Input: dimensioned drawing with shaded views. Units: mm. Origin: part minimum x, y, z. A direction names the side the tool comes from. Coordinates: 2 decimals unless noted, no trailing zeros. Loops run counter-clockwise (first coordinate to the right, second up) from the corner with the lowest first, then second, coordinate; pieces in that order, holes last.
Item 1: Line query: probe 1 along Z at (x, y) = (18.75, 20.5) (1 decimal); probe 2 along Y at (x, z) = (10.25, 5.5) (1 decimal); probe 3 along Z at (x, y) = (12.7, 1.4). Output: solid intervals per line, ascending.
Item 2: Section query B-B, the plane y = 12.7. Return the cut outline in (x, z) (1 decimal).
Item 3: Pin query (flat end, axial travel): pin 1 Ø12 at (x, z) = (7.5, 3.5) entering from +Y (3 decimals); pin 2 Ø13.5 at (x, y) = (14, 15) entering from -Z (3 decimals); pin 3 Ø1 at (x, y) = (9, 5) entering from -Z (1 decimal). Return the tip coordinate at first contact, or that it passes through.
Item 4: Reachability of the marked faces 3 and 4 from +Z, -Z, +X, -X, +Y, -Y: full face, straight path, thin tool, end or side. Return the list, or none.
Item 5: Section query C-C, the plane z = 13.5. Return the cut outline in (x, y) (1 decimal), then the cut area to 3 significant figures.
Item 6: Pull-direction query (X, two-part tool) for the marked faces 1 and 2; classes: +X half, -X half, draft (parallel to the pull), parting line (faces both ways), or undercut.
Item 7: Section query A-A, the plane x = 12.7. Return the cut outline in (y, z) (1 decimal), then the cut area to 3 significant figures.
Item 8: Section query D-D, the plane x = 22.25. Return the cut outline in (y, z) (1 decimal).
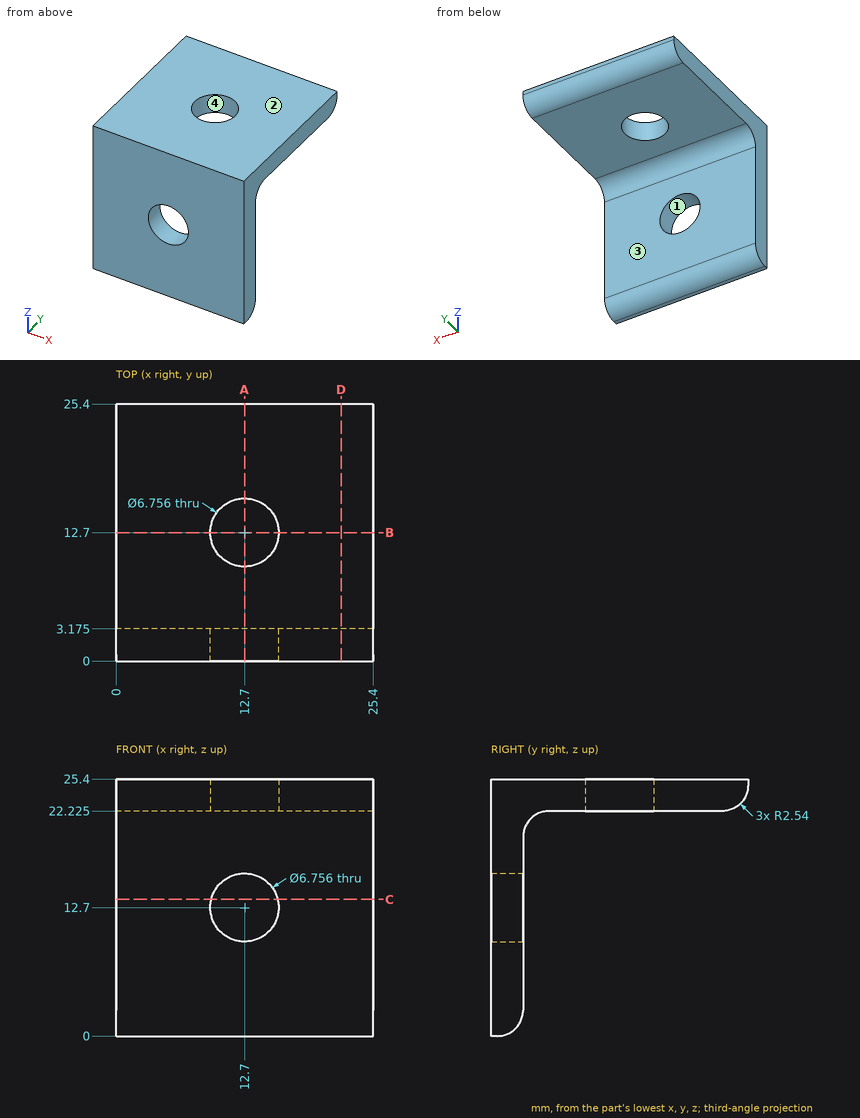
Verdict:
1. probe 1: z = 22.2 to 25.4
1. probe 2: y = 0 to 3.2
1. probe 3: z = 0.12 to 9.32, 16.08 to 25.4
2. outline: (0, 22.2) - (9.3, 22.2) - (9.3, 25.4) - (0, 25.4) - close; (16.1, 22.2) - (25.4, 22.2) - (25.4, 25.4) - (16.1, 25.4) - close
3. pin 1: stops at y = 3.175
3. pin 2: stops at z = 22.225
3. pin 3: stops at z = 21.9
4. face 3: -Z, +X, -X, +Y
4. face 4: +Z, -Z
5. outline: (0, 0) - (9.4, 0) - (9.4, 3.2) - (0, 3.2) - close; (16, 0) - (25.4, 0) - (25.4, 3.2) - (16, 3.2) - close
5. area: 59.8 mm2
6. face 1: undercut
6. face 2: draft
7. outline: (0, 0) - (0.6, 0) arc R2.5 ccw to (3.2, 2.5) - (3.2, 9.3) - (0, 9.3) - close; (0, 16.1) - (3.2, 16.1) - (3.2, 19.7) arc R2.5 cw to (5.7, 22.2) - (9.3, 22.2) - (9.3, 25.4) - (0, 25.4) - close; (16.1, 22.2) - (22.9, 22.2) arc R2.5 ccw to (25.4, 24.8) - (25.4, 25.4) - (16.1, 25.4) - close
7. area: 107 mm2
8. outline: (0, 0) - (0.6, 0) arc R2.5 ccw to (3.2, 2.5) - (3.2, 19.7) arc R2.5 cw to (5.7, 22.2) - (22.9, 22.2) arc R2.5 ccw to (25.4, 24.8) - (25.4, 25.4) - (0, 25.4) - close
